Model file for the job. Use its own axes, mm. A direction names the side the tool comes from. Give positions to 0.01 mm unless a question says otherwise; leave off trailing zeros. Order: outer loops, then holes, each group sorted by start corner. A loop starts at its lowest first (then second) coordinate and runs counter-clockwise, first axis right, second up. Notation, with made-up numbers: (86.5, 32) -> (141.5, 32) arc R11 cw to (141.5, 52) -> close; hole circle Ø5 at (75.25, 1.25). An arc over 180 degrees is marked (long way). Use CSV: the item, a comma, the result in double quotes. Start each with the question number.
1. Wall check: line 1 (X direction, y = 3.25, z = 2); line 2 (Z direction, x = -1, y = 2); line 3 (Y direction, x = 4, z = 0.79). Give the ranges that are in metal, low to high. Write a range as from..to.
2. Cut at D-D on y = 2.75. List the corners of the cut face in (x, z), then the cut area to 3 significant figures.
3. Cut at C-C on y = -1.5. List the corners of the cut face in (x, z).
4. Cut at B-B on z = 2.75. List the corners of the cut face in (x, y).
5. Cut at A-A on x = 2. List the corners of the cut face in (y, z).
6. 3-axis set-ups, long thin cutter, end or side, ignore diameter. For faces 4 (the flat face through (3.131, -3.437, -1.917)), 5 (the flat face through (0, 3.1, 2.1)): which of +Z, -Z, +X, -X, +Y, -Y reach the whole face in a straight line?
7. Drop a flat-ended pin along its axis: pin 1 (1.5 mm diameter, centred on x = 3.5, z = 1, fed in from +Y). Give the stop position or say it passes through.
8. Pull direction Y, two halves, no side cores. Call faces 1 (the flat face through (6.35, -1, -2)), 2 (the cylindrical face through (2.49, -2.44, 0.25)), 3 (the cylindrical face through (-0.626, 1.072, 3.405)): released by +Y, released by -Y, zero draft, split by the parting line, or undercut.
```python
from build123d import *

# Parameters (mm, degrees)
BOSS_EXTRUDE1_DEPTH = 6.35
SKETCH4_R           = 3.57
BOSS_EXTRUDE2_DEPTH = 1.27
SKETCH3_R           = 2.5
CUT_EXTRUDE1_DEPTH  = 8.62
SKETCH5_R           = 1
CUT_EXTRUDE3_DEPTH  = 0.15


with BuildPart() as part:
    # Sketch2 → Boss-Extrude1 (new body)
    with BuildSketch(Plane(origin=(0, 0, 0), x_dir=(0, 0, -1), z_dir=(1, 0, 0))):
        Polygon((3.919437566, -2.29861752), (3.950379949, 2.245023741), (0.030942383, 4.54364126), (-3.919437566, 2.29861752), (-3.950379949, -2.245023741), (-0.030942383, -4.54364126), align=None)
    extrude(amount=BOSS_EXTRUDE1_DEPTH)

    # Sketch4 → Boss-Extrude2 (add)
    with BuildSketch(Plane.ZY):
        Circle(SKETCH4_R)
    extrude(amount=BOSS_EXTRUDE2_DEPTH)

    # Sketch3 → Cut-Extrude1 (cut, through all)
    with BuildSketch(Plane.ZY.offset(1.27)):
        with Locations((0.79, 0)):
            Circle(SKETCH3_R)
    extrude(amount=-CUT_EXTRUDE1_DEPTH, mode=Mode.SUBTRACT)

    # Sketch5 → Cut-Extrude3 (cut)
    with BuildSketch(Plane(origin=(0, 0.02679689, 3.934908757), x_dir=(1, 0, 0), z_dir=(0, -0.006809883, -0.999976812))):
        with Locations((3.175, 0)):
            Circle(SKETCH5_R)
    extrude(amount=CUT_EXTRUDE3_DEPTH, mode=Mode.SUBTRACT)


solid = part.part
```
Verdict:
1,line 1,"0..6.35"
1,line 2,"-2.96..-0.71, 2.29..2.96"
1,line 3,"-4.1..-2.5, 2.5..4.08"
2,outline,"(-1.27, -2.28) -> (0, -2.28) -> (0, -3.09) -> (6.35, -3.09) -> (6.35, 3.13) -> (0, 3.13) -> (0, 2.28) -> (-1.27, 2.28) -> close"
2,area,"45.2 mm^2"
3,outline,"(-1.27, -3.24) -> (0, -3.24) -> (0, -3.92) -> (6.35, -3.92) -> (6.35, -1.21) -> (-1.27, -1.21) -> close; (-1.27, 2.79) -> (6.35, 2.79) -> (6.35, 3.95) -> (0, 3.95) -> (0, 3.24) -> (-1.27, 3.24) -> close"
4,outline,"(-1.27, -2.28) -> (0, -2.28) -> (0, -2.95) -> (6.35, -2.95) -> (6.35, -1.55) -> (-1.27, -1.55) -> close; (-1.27, 1.55) -> (6.35, 1.55) -> (6.35, 2.96) -> (0, 2.96) -> (0, 2.28) -> (-1.27, 2.28) -> close"
5,outline,"(-4.54, 0.03) -> (-2.3, -3.92) -> (2.25, -3.95) -> (4.54, -0.03) -> (2.3, 3.92) -> (-2.25, 3.95) -> close; hole circle Ø5 at (0, 0.79)"
6,face 4,"-Z, +X, -X, -Y"
6,face 5,"-X"
7,pin 1,"y = 4.38"
8,face 1,"zero draft"
8,face 2,"undercut"
8,face 3,"split by the parting line"
